Source: CAD feature listing. Evaluate the final solid. Frame: model axes, mm. A direction names the side the tool comes from. Give positions to 0.01 mm unless a question says otherwise; leave off trailing zeros. Write each loop counter-clockwise with the first axis right and the second up, starting at its lowest first coordinate (ties: lowest second). Pieces come first, ordered by that corner, then holes. Notation, with made-up numbers: (-38, 75) - (-19, 75) arc R30 cw to (-19, 101) - close; hole circle Ø8 at (-3.5, 39). An arc over 180 degrees is marked (long way). One line per question, with ' | ' between items. Start each with the question number.
(1) Section B-B, the plane y = 9.75. State how many separate pieces and enclosed holes the cut face has, plus the area to 3 significant figures.
(2) Section A-A, the plane x = 0. Return loops of the section in (y, z) (3 decimals).
(3) Draft query along Z for faces 1 (the flat face through (-12.95, 12.52, -11.18)), 2 (the flat face through (0, 7, -51.912)). Return one class per face: +Z half, -Z half, draft (parallel to the pull), parting line (faces both ways), or undercut.
(4) Ray query, line 1 (Z direction, x = 1, y = 1.5); line 2 (X direction, y = 11.75, z = 10); line 3 (Z direction, x = -3, y = 12.5). Return the intervals inside material, ascending. Write a range as [from, to].
(5) Access query for faces 3 (the flat face through (-9.703, 12.521, -7.456)), 4 (the cylindrical face through (8.505, 5.423, 10.33)), 5 (the flat face through (-0.2, 10.5, -7.2)). Directions: +Z, -Z, +X, -X, +Y, -Y. A direction counts if a zero-diameter tool reaches every point of the face in a straight line with its end or side. Return the directions, or none.
(6) Pin query (flat end, axial travel): pin 1 (3 mm diameter, centred on x = -10.25, z = 10.25, fed in from -Y); pin 2 (18 mm diameter, centred on x = 0, z = 0, fed in from +Y); pin 3 (1 mm diameter, centred on x = 4.5, y = 9, fed in from +Z); pin 4 (1 mm diameter, centred on x = 6.5, y = 4.5, fed in from -Z). Return the tip coordinate at first contact, or that it passes through.
```python
from build123d import *

# Parameters (mm, degrees)
SKETCH1_R           = 7
BOSS_EXTRUDE1_DEPTH = 14
SKETCH2_R           = 11.075
CUT_EXTRUDE1_DEPTH  = 10.5
SKETCH4_R           = 1.75
CUT_EXTRUDE4_DEPTH  = 15
CUT_EXTRUDE5_DEPTH  = 3
SKETCH6_R           = 3.25
CUT_EXTRUDE6_DEPTH  = 15
SKETCH7_R           = 5.5
CUT_EXTRUDE7_DEPTH  = 5
FILLET4_R           = 6


with BuildPart() as part:
    # Sketch1 → Boss-Extrude1 (new body)
    with BuildSketch(Plane(origin=(0, 0, 0), x_dir=(1, 0, 0), z_dir=(0, 1, 0))):
        with BuildLine():
            Line((-7.5, 51.911534525), (7.5, 51.911534525))
            Line((7.5, 51.911534525), (13.985690309, 12.109932558))
            ThreePointArc((13.985690309, 12.109932558), (0, -18.5), (-13.985690309, 12.109932558))
            Line((-13.985690309, 12.109932558), (-7.5, 51.911534525))
        make_face()
        Circle(SKETCH1_R, mode=Mode.SUBTRACT)
    extrude(amount=BOSS_EXTRUDE1_DEPTH)

    # Sketch2 → Cut-Extrude1 (cut)
    with BuildSketch(Plane.XZ):
        Circle(SKETCH2_R)
    extrude(amount=-CUT_EXTRUDE1_DEPTH, mode=Mode.SUBTRACT)

    # Sketch4 → Cut-Extrude4 (cut, through all)
    with BuildSketch(Plane.XZ):
        with Locations((10.253048327, 10.253048327)):
            Circle(SKETCH4_R)
        with Locations((10.253048327, -10.253048327)):
            Circle(SKETCH4_R)
        with Locations((-10.253048327, -10.253048327)):
            Circle(SKETCH4_R)
        with Locations((-10.253048327, 10.253048327)):
            Circle(SKETCH4_R)
    extrude(amount=-CUT_EXTRUDE4_DEPTH, mode=Mode.SUBTRACT)

    # Sketch5 → Cut-Extrude5 (cut)
    with BuildSketch(Plane(origin=(0, 14, 0), x_dir=(1, 0, 0), z_dir=(0, 1, 0))):
        Polygon((13.375361377, 9.2132593), (12.714688564, 12.437156233), (9.592375514, 13.47694526), (7.130735278, 11.292837354), (7.79140809, 8.068940421), (10.91372114, 7.029151394), align=None)
        Polygon((-9.2132593, 13.375361377), (-12.437156233, 12.714688564), (-13.47694526, 9.592375514), (-11.292837354, 7.130735278), (-8.068940421, 7.79140809), (-7.029151394, 10.91372114), align=None)
        Polygon((9.2132593, -13.375361377), (12.437156233, -12.714688564), (13.47694526, -9.592375514), (11.292837354, -7.130735278), (8.068940421, -7.79140809), (7.029151394, -10.91372114), align=None)
        Polygon((-13.375361377, -9.2132593), (-12.714688564, -12.437156233), (-9.592375514, -13.47694526), (-7.130735278, -11.292837354), (-7.79140809, -8.068940421), (-10.91372114, -7.029151394), align=None)
    extrude(amount=-CUT_EXTRUDE5_DEPTH, mode=Mode.SUBTRACT)

    # Sketch6 → Cut-Extrude6 (cut, through all)
    with BuildSketch(Plane(origin=(0, 14, 0), x_dir=(1, 0, 0), z_dir=(0, 1, 0))):
        with Locations((0, 44.911534525)):
            Circle(SKETCH6_R)
        with Locations((0, 28.911534525)):
            Circle(SKETCH6_R)
    extrude(amount=-CUT_EXTRUDE6_DEPTH, mode=Mode.SUBTRACT)

    # Sketch7 → Cut-Extrude7 (cut)
    with BuildSketch(Plane(origin=(0, 14, 0), x_dir=(1, 0, 0), z_dir=(0, 1, 0))):
        with Locations((0, 28.911534525)):
            Circle(SKETCH7_R)
        with Locations((0, 44.911534525)):
            Circle(SKETCH7_R)
    extrude(amount=-CUT_EXTRUDE7_DEPTH, mode=Mode.SUBTRACT)

    # Fillet4
    fillet4_edges = [part.edges().sort_by_distance(p)[0] for p in [
        (-7.5, 7, -51.911534525),
        (7.5, 7, -51.911534525),
        (13.985690309, 7, -12.109932558),
        (-13.985690309, 7, -12.109932558),
    ]]
    fillet(fillet4_edges, radius=FILLET4_R)


solid = part.part
```
Check sheet entries:
1) separate pieces: 1 | enclosed holes: 7 | area: 1,180 mm²
2) outline: (0, -51.912) - (14, -51.912) - (14, -50.412) - (9, -50.412) - (9, -48.162) - (0, -48.162) - close; (0, -41.662) - (9, -41.662) - (9, -39.412) - (14, -39.412) - (14, -34.412) - (9, -34.412) - (9, -32.162) - (0, -32.162) - close; (0, -25.662) - (9, -25.662) - (9, -23.412) - (14, -23.412) - (14, -7) - (10.5, -7) - (10.5, -11.075) - (0, -11.075) - close; (0, 11.075) - (10.5, 11.075) - (10.5, 7) - (14, 7) - (14, 18.5) - (0, 18.5) - close
3) face 1: undercut | face 2: -Z half
4) line 1: [-51.91, -48], [-41.82, -32], [-25.82, -11.03], [11.03, 18.47] | line 2: [-15.56, -13.21], [-7.4, 7.33], [13.34, 15.56] | line 3: [-51.88, -49.52], [-40.3, -33.52], [-24.3, -6.32], [6.32, 18.26]
5) face 3: +Y | face 4: +Y, -Y | face 5: -Y
6) pin 1: through | pin 2: y = 14 | pin 3: z = 18.06 | pin 4: z = -50.71
